Geometry check sheet. Reference: drawing and pictorial views, mm from the part's lowest x, y, z. A direction names the side the tool comes from. Give positions to 0.01 mm unless a question says otherwise; leave off trailing zeros. Order: outer loops, then holes, each group sorted by start corner. A loop starts at its lowest first (then second) coordinate and runs counter-clockwise, first axis right, second up. Notation, with made-up numbers: (-29, 14.25) - (22, 14.25) arc R3 ccw to (22, 18.25) - close; hole circle Ø1 at (20, 67.25). An arc over 180 degrees is marked (long way). Answer in a Markdown table with one row per item.
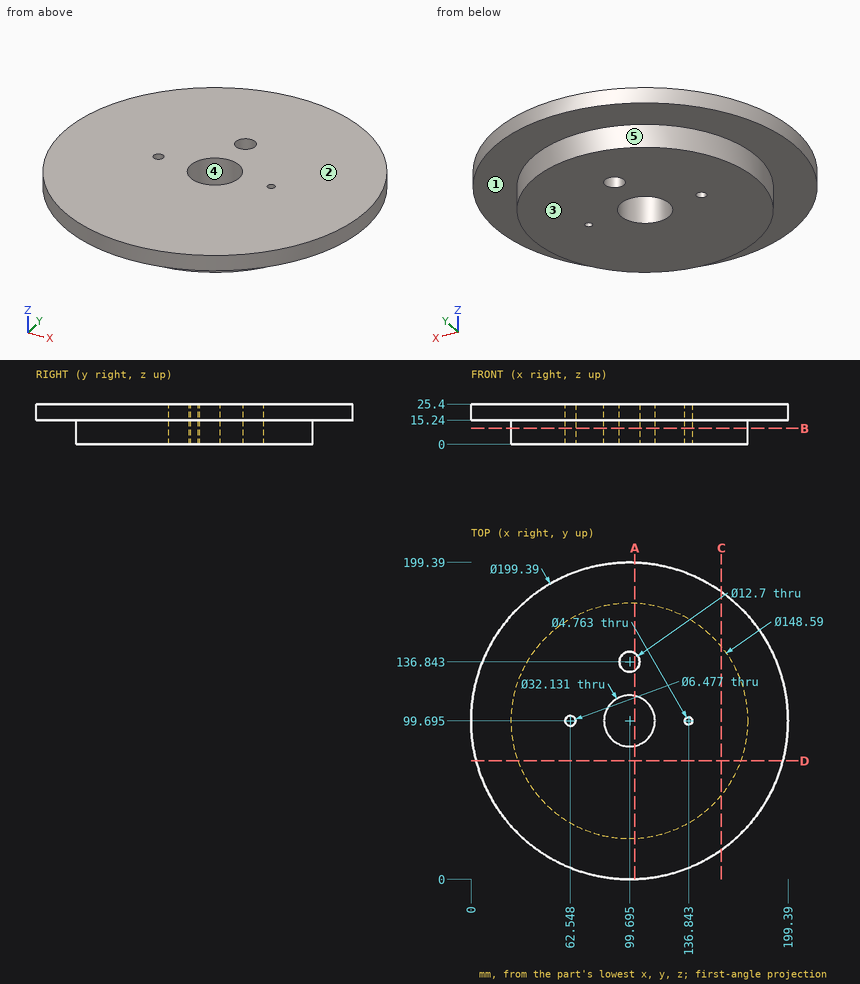
(1) Mould release check, pull along X, two halves, no side actions. Record for the marked faces 3, 4 and 5: pulls with the +X half, pulls with the -X half, needs draft (parallel to the pull), parting line crosses it, or undercut.
Geometry says:
| item | result |
|---|---|
| face 3 | needs draft |
| face 4 | undercut |
| face 5 | parting line crosses it |
(2) Cross-section at D-D, the plane y = 74.5. Record the cut outline in (x, z), then the cut area to 3 significant figures.
Geometry says:
| item | result |
|---|---|
| outline | (3.24, 15.24) - (29.8, 15.24) - (29.8, 0) - (169.59, 0) - (169.59, 15.24) - (196.15, 15.24) - (196.15, 25.4) - (3.24, 25.4) - close |
| area | 4,090 mm² |
(3) Cross-section at A-A, the plane x = 103. Record the cut outline in (y, z) (1 decimal).
Geometry says:
| item | result |
|---|---|
| outline | (0.1, 15.2) - (25.5, 15.2) - (25.5, 0) - (84, 0) - (84, 25.4) - (0.1, 25.4) - close; (115.4, 0) - (131.4, 0) - (131.4, 25.4) - (115.4, 25.4) - close; (142.3, 0) - (173.9, 0) - (173.9, 15.2) - (199.3, 15.2) - (199.3, 25.4) - (142.3, 25.4) - close |
(4) Thickness scan on L1, parallel to Z at x = 175.5, y = 46.5; L2, parallel to X at y = 132, z = 22 (1 decimal); L3, parallel to X at y = 90, z = 3.75 (1 decimal). Record the ranges inside material, lowest first.
Geometry says:
| item | result |
|---|---|
| L1 | 15.24 to 25.4 |
| L2 | 5.4 to 95.6, 103.8 to 194 |
| L3 | 26 to 86.9, 112.5 to 173.4 |
(5) Cross-section at B-B, the plane z = 10. Give the number of separate pieces and of enclosed holes in the cut face, then the cut area to 3 significant figures.
Geometry says:
| item | result |
|---|---|
| separate pieces | 1 |
| enclosed holes | 4 |
| area | 16,400 mm² |
(6) Gauge pin test, flat ends, axial feed: P1, Ø1, axis at x = 93, z = 17, coming from the -Y side; P2, Ø12, axis at y = 151.5, z = 21, coming from the +X side (1 decimal); P3, Ø8, axis at y = 28, z = 17.5, coming from the -X side. Record the tip position at first contact, or that the pin passes through.
Geometry says:
| item | result |
|---|---|
| P1 | y = 0.19 |
| P2 | x = 188.2 |
| P3 | x = 26.51 |
(7) Cross-section at C-C, the plane x = 157.5. Record the cut outline in (y, z), then the cut area to 3 significant figures.
Geometry says:
| item | result |
|---|---|
| outline | (18.47, 15.24) - (53.02, 15.24) - (53.02, 0) - (146.37, 0) - (146.37, 15.24) - (180.92, 15.24) - (180.92, 25.4) - (18.47, 25.4) - close |
| area | 3,070 mm² |
(8) Access from +Z, -Z, +X, -X, +Y, -Y to the whole of each face (thin tool, end or side, straight path). Record for the marked faces 1 and 2.
Geometry says:
| item | result |
|---|---|
| face 1 | -Z |
| face 2 | +Z, +X, -X, +Y, -Y |
